from build123d import *

# Parameters (mm, degrees)
SKETCH_1_R          = 2.5
EXTRUDE_1_DEPTH     = 300
SKETCH_2_R          = 1.75
CUT_EXTRUDE_1_DEPTH = 39


with BuildPart() as part:
    # 草图1 → 凸台-拉伸1 (new body)
    with BuildSketch(Plane.XY):
        with BuildLine():
            Line((-4.415608984, 3.873972711), (-4.415608984, -1.204706946))
            Line((-4.415608984, -1.204706946), (-7.376269156, -4.165367117))
            Line((-7.376269156, -4.165367117), (-9.015608984, -4.165367117))
            Line((-9.015608984, -4.165367117), (-9.015608984, -1.765367117))
            Line((-9.015608984, -1.765367117), (-10.015608984, -1.765367117))
            Line((-10.015608984, -1.765367117), (-10.015608984, -2.265367117))
            Line((-10.015608984, -2.265367117), (-10.815608984, -2.265367117))
            Line((-10.815608984, -2.265367117), (-10.815608984, -7.165367117))
            ThreePointArc((-10.815608984, -7.165367117), (-10.376269156, -8.226027289), (-9.315608984, -8.665367117))
            Line((-9.315608984, -8.665367117), (-4.415608984, -8.665367117))
            Line((-4.415608984, -8.665367117), (-4.415608984, -7.865367117))
            Line((-4.415608984, -7.865367117), (-3.915608984, -7.865367117))
            Line((-3.915608984, -7.865367117), (-3.915608984, -6.865367117))
            Line((-3.915608984, -6.865367117), (-6.315608984, -6.865367117))
            Line((-6.315608984, -6.865367117), (-6.315608984, -5.226027289))
            Line((-6.315608984, -5.226027289), (-3.354948812, -2.265367117))
            Line((-3.354948812, -2.265367117), (1.723730844, -2.265367117))
            Line((1.723730844, -2.265367117), (4.684391016, -5.226027289))
            Line((4.684391016, -5.226027289), (4.684391016, -6.865367117))
            Line((4.684391016, -6.865367117), (2.284391016, -6.865367117))
            Line((2.284391016, -6.865367117), (2.284391016, -7.865367117))
            Line((2.284391016, -7.865367117), (2.784391016, -7.865367117))
            Line((2.784391016, -7.865367117), (2.784391016, -8.665367117))
            Line((2.784391016, -8.665367117), (7.684391016, -8.665367117))
            ThreePointArc((7.684391016, -8.665367117), (8.745051188, -8.226027289), (9.184391016, -7.165367117))
            Line((9.184391016, -7.165367117), (9.184391016, -2.265367117))
            Line((9.184391016, -2.265367117), (8.384391016, -2.265367117))
            Line((8.384391016, -2.265367117), (8.384391016, -1.765367117))
            Line((8.384391016, -1.765367117), (7.384391016, -1.765367117))
            Line((7.384391016, -1.765367117), (7.384391016, -4.165367117))
            Line((7.384391016, -4.165367117), (5.745051188, -4.165367117))
            Line((5.745051188, -4.165367117), (2.784391016, -1.204706946))
            Line((2.784391016, -1.204706946), (2.784391016, 3.873972711))
            Line((2.784391016, 3.873972711), (5.745051188, 6.834632883))
            Line((5.745051188, 6.834632883), (7.384391016, 6.834632883))
            Line((7.384391016, 6.834632883), (7.384391016, 4.434632883))
            Line((7.384391016, 4.434632883), (8.384391016, 4.434632883))
            Line((8.384391016, 4.434632883), (8.384391016, 4.934632883))
            Line((8.384391016, 4.934632883), (9.184391016, 4.934632883))
            Line((9.184391016, 4.934632883), (9.184391016, 9.834632883))
            ThreePointArc((9.184391016, 9.834632883), (8.745051188, 10.895293054), (7.684391016, 11.334632883))
            Line((7.684391016, 11.334632883), (2.784391016, 11.334632883))
            Line((2.784391016, 11.334632883), (2.784391016, 10.534632883))
            Line((2.784391016, 10.534632883), (2.284391016, 10.534632883))
            Line((2.284391016, 10.534632883), (2.284391016, 9.534632883))
            Line((2.284391016, 9.534632883), (4.684391016, 9.534632883))
            Line((4.684391016, 9.534632883), (4.684391016, 7.895293054))
            Line((4.684391016, 7.895293054), (1.723730844, 4.934632883))
            Line((1.723730844, 4.934632883), (-3.354948812, 4.934632883))
            Line((-3.354948812, 4.934632883), (-6.315608984, 7.895293054))
            Line((-6.315608984, 7.895293054), (-6.315608984, 9.534632883))
            Line((-6.315608984, 9.534632883), (-3.915608984, 9.534632883))
            Line((-3.915608984, 9.534632883), (-3.915608984, 10.534632883))
            Line((-3.915608984, 10.534632883), (-4.415608984, 10.534632883))
            Line((-4.415608984, 10.534632883), (-4.415608984, 11.334632883))
            Line((-4.415608984, 11.334632883), (-9.315608984, 11.334632883))
            ThreePointArc((-9.315608984, 11.334632883), (-10.376269156, 10.895293054), (-10.815608984, 9.834632883))
            Line((-10.815608984, 9.834632883), (-10.815608984, 4.934632883))
            Line((-10.815608984, 4.934632883), (-10.015608984, 4.934632883))
            Line((-10.015608984, 4.934632883), (-10.015608984, 4.434632883))
            Line((-10.015608984, 4.434632883), (-9.015608984, 4.434632883))
            Line((-9.015608984, 4.434632883), (-9.015608984, 6.834632883))
            Line((-9.015608984, 6.834632883), (-7.376269156, 6.834632883))
            Line((-7.376269156, 6.834632883), (-4.415608984, 3.873972711))
        make_face()
        with Locations((-0.815608984, 1.334632883)):
            Circle(SKETCH_1_R, mode=Mode.SUBTRACT)
    extrude(amount=EXTRUDE_1_DEPTH)

    # 草图2 → 切除-拉伸1 (cut)
    with BuildSketch(Plane(origin=(2.784391016, 0, 0), x_dir=(0, 0, -1), z_dir=(1, 0, 0))):
        with Locations(Location((-250, 1.334632883, 0), (0, 0, 90))):
            Circle(SKETCH_2_R)
        with Locations(Location((-50, 1.334632883, 0), (0, 0, 90))):
            Circle(SKETCH_2_R)
    extrude(amount=-CUT_EXTRUDE_1_DEPTH, mode=Mode.SUBTRACT)


solid = part.part
Read the model definition and answer for the solid it produces. Units are mm, in the model's axes. A direction names the side the tool comes from. Round coordinates to 2 decimals unless told otherwise and drop trailing zeros. One line per question, with ' | ' between items. Start each with the question number.
Q1. For a pull along Y with two mould halves and no side action, classify faces 1 (the flat face through (-1, -2.265, 148)), 2 (the flat face through (-4.416, 1, 148)), 3 (the cylindrical face through (1.569, 2.086, 147.9)), 4 (the flat face through (-10.816, 7, 148)) as +Y half, -Y half, draft (parallel to the pull), parting line (faces both ways), or undercut.
Q2. Flat-ended cylindrical pins translate along their axes: pin 1 (0.5 mm diameter, centred on x = 8, z = 160, fed in from -Y); pin 2 (1.5 mm diameter, centred on x = -1.5, z = 208.5, fed in from -Y); pin 3 (5.5 mm diameter, centred on y = 1.5, z = 181, fed in from -X); pin 4 (5.5 mm diameter, centred on x = 0, z = 77, fed in from +Y). Find the tip coordinate at first contact, or state that the pin passes through.
Q3. Find the intervals of material crossed by L1, parallel to Y at x = 1.7, z = 50; L2, parallel to X at y = 9, z = 181.5; L3, parallel to X at y = -3.5, z = 267, in increasing order.
Q4. For faces 5 (the flat face through (-1, 4.935, 148)), 6 (the flat face through (2.784, 1, 148)), 7 (the flat face through (-3, 4, 300)), determine the directions among +Z, -Z, +X, -X, +Y, -Y from which every point of the face is accessible in a straight line to the end or side of a thin tool.
Established:
1) face 1: -Y half | face 2: undercut | face 3: undercut | face 4: draft
2) pin 1: y = -8.66 | pin 2: y = -2.27 | pin 3: x = -4.79 | pin 4: y = 10.53
3) L1: -2.27 to -0.42, 3.08 to 4.93 | L2: -10.82 to -6.32, 4.68 to 9.18 | L3: -10.82 to -9.02, -6.71 to -4.59, 2.96 to 5.08, 7.38 to 9.18
4) face 5: +Z, -Z, +Y | face 6: +Z, -Z, +X | face 7: +Z, +X, -X, +Y, -Y
